Geometry: final body of the model. Coordinates: model frame, mm. A direction names the side the tool comes from. Give positions to 0.01 mm unless a question says otherwise; leave off trailing zeros. Loops run counter-clockwise (first coordinate to the right, second up) from the corner with the lowest first, then second, coordinate; pieces in that order, holes last. Notation, with made-up numbers: (-10.5, 65.5) - (42.5, 65.5) arc R19 ccw to (42.5, 101.5) - close; hole circle Ø5 at (-11.75, 54). An arc over 180 degrees is marked (long way). Use one line per item in the form item = value.
```python
from build123d import *

# Parameters (mm, degrees)
F0_W     = 6.35
F0_H     = 78.9432
F0_R     = 1.7145
F0_H_2   = 35.56
F1_DEPTH = 6.35
F2_DEPTH = 8.255


with BuildPart() as f1:
    # F0 (on Front) → F1 (new body)
    with BuildSketch(Plane.XZ):
        with Locations((-53.975, 30.3784)):
            Rectangle(F0_W, F0_H)
        with Locations((-53.975, -4.9657)):
            Circle(F0_R, mode=Mode.SUBTRACT)
        with Locations((-53.975, 65.7225)):
            Circle(F0_R, mode=Mode.SUBTRACT)
        with Locations((-53.975, -52.07)):
            Rectangle(F0_W, F0_H_2)
        with Locations((-53.975, -65.7225)):
            Circle(F0_R, mode=Mode.SUBTRACT)
        with Locations((-53.975, -38.4175)):
            Circle(F0_R, mode=Mode.SUBTRACT)
        with Locations((53.975, -52.07)):
            Rectangle(F0_W, F0_H_2)
        with Locations((53.975, -65.7225)):
            Circle(F0_R, mode=Mode.SUBTRACT)
        with Locations((53.975, -38.4175)):
            Circle(F0_R, mode=Mode.SUBTRACT)
        with Locations((53.975, 30.3784)):
            Rectangle(F0_W, F0_H)
        with Locations((53.975, -4.9657)):
            Circle(F0_R, mode=Mode.SUBTRACT)
        with Locations((53.975, 65.7225)):
            Circle(F0_R, mode=Mode.SUBTRACT)
        Polygon((-47.625, -69.85), (47.625, -69.85), (47.625, -31.115), (57.15, -31.115), (57.15, -12.2682), (47.625, -12.2682), (47.625, 69.85), (28.575, 69.85), (28.575, 31.75), (-28.575, 31.75), (-28.575, 69.85), (-47.625, 69.85), (-47.625, -12.2682), (-57.15, -12.2682), (-57.15, -31.115), (-47.625, -31.115), align=None)
        Polygon((-14.605, 15.875), (-14.605, 19.05), (-8.255, 19.05), (-8.255, 15.875), (-8.255, -38.2016), (-8.255, -41.3766), (-14.605, -41.3766), (-14.605, -38.2016), align=None, mode=Mode.SUBTRACT)
        Polygon((8.255, 15.875), (8.255, 19.05), (14.605, 19.05), (14.605, 15.875), (14.605, -38.2016), (14.605, -41.3766), (8.255, -41.3766), (8.255, -38.2016), align=None, mode=Mode.SUBTRACT)
    extrude(amount=F1_DEPTH)

    # F0 (on Front) → F2 (join)
    with BuildSketch(Plane.XZ):
        Polygon((47.625, -12.2682), (57.15, -12.2682), (57.15, -9.0932), (50.8, -9.0932), (50.8, 69.85), (47.625, 69.85), align=None)
        Polygon((47.625, -69.85), (50.8, -69.85), (50.8, -34.29), (57.15, -34.29), (57.15, -31.115), (47.625, -31.115), align=None)
        Polygon((-57.15, -9.0932), (-57.15, -12.2682), (-47.625, -12.2682), (-47.625, 69.85), (-50.8, 69.85), (-50.8, -9.0932), align=None)
        Polygon((-50.8, -69.85), (-47.625, -69.85), (-47.625, -31.115), (-57.15, -31.115), (-57.15, -34.29), (-50.8, -34.29), align=None)
    extrude(amount=F2_DEPTH)


solid = f1.part
```
(1) Cut plane A-A (z = 8). Return the cut outline in (x, y) (3 decimals), plus the area to 3 significant figures.
Solution:
outline = (-57.15, -6.35) - (-50.8, -6.35) - (-50.8, -8.255) - (-47.625, -8.255) - (-47.625, -6.35) - (-14.605, -6.35) - (-14.605, 0) - (-57.15, 0) - close; (-8.255, -6.35) - (8.255, -6.35) - (8.255, 0) - (-8.255, 0) - close; (14.605, -6.35) - (47.625, -6.35) - (47.625, -8.255) - (50.8, -8.255) - (50.8, -6.35) - (57.15, -6.35) - (57.15, 0) - (14.605, 0) - close
area = 657 mm2
(2) Access query for faces 1 (the face through (0, -3, 31.75)), 2 (the face through (11, -3, -41.377)), 3 (the face through (-54, -6.35, 31)). Directions: +Z, -Z, +X, -X, +Y, -Y. A direction counts if a zero-diameter tool reaches every point of the face in a straight line with its end or side. Return the directions, or none.
Solution:
face_1 = +Z, +Y, -Y
face_2 = +Y, -Y
face_3 = +Z, -X, -Y
(3) Material intervals for L1, parallel to X at y = -5.75, z = -1 (3 decimals); L2, parallel to X at y = -1, z = -5 (3 decimals); L3, parallel to X at y = -7.5, z = 15 (3 decimals), sorted ascending. Write a range as from..to.
Solution:
L1 = -57.15..-14.605, -8.255..8.255, 14.605..57.15
L2 = -57.15..-55.689, -52.261..-14.605, -8.255..8.255, 14.605..52.261, 55.689..57.15
L3 = -50.8..-47.625, 47.625..50.8
(4) Pin query (flat end, axial travel): P1, Ø4.5, axis at x = 53.98, z = 65.72, coming from the -Y side; P2, Ø6, axis at x = -31, z = 48, coming from the +Y side; P3, Ø0.6, axis at y = -7, z = -55, coming from the +X side; P4, Ø2, axis at x = 54, y = -7.5, coming from the +Z side. Return the tip coordinate at first contact, or that it passes through.
Solution:
P1 = -6.35
P2 = 0
P3 = 50.8
P4 = -9.09
(5) Cut plane B-B (x = -10.5). Return the cut outline in (y, z).
Solution:
outline = (-6.35, -69.85) - (0, -69.85) - (0, -41.38) - (-6.35, -41.38) - close; (-6.35, 19.05) - (0, 19.05) - (0, 31.75) - (-6.35, 31.75) - close
(6) Pull-direction query (Z, two-part tool) for faces 4 (the face through (-1, -3, -69.85)), 5 (the face through (54.897, -3.131, 67.168)), 6 (the face through (-50, -8.255, 26)); classes: released by +Z, released by -Z, zero draft, split by the parting line, or undercut.
Solution:
face_4 = released by -Z
face_5 = undercut
face_6 = zero draft
(7) Cut plane D-D (z = -55). Return the cut outline in (x, y) (3 decimals).
Solution:
outline = (-57.15, -6.35) - (-50.8, -6.35) - (-50.8, -8.255) - (-47.625, -8.255) - (-47.625, -6.35) - (47.625, -6.35) - (47.625, -8.255) - (50.8, -8.255) - (50.8, -6.35) - (57.15, -6.35) - (57.15, 0) - (-57.15, 0) - close
(8) Cut plane C-C (z = 43.5). Return the cut outline in (x, y) (3 decimals), plus the area to 3 significant figures.
Solution:
outline = (-57.15, -6.35) - (-50.8, -6.35) - (-50.8, -8.255) - (-47.625, -8.255) - (-47.625, -6.35) - (-28.575, -6.35) - (-28.575, 0) - (-57.15, 0) - close; (28.575, -6.35) - (47.625, -6.35) - (47.625, -8.255) - (50.8, -8.255) - (50.8, -6.35) - (57.15, -6.35) - (57.15, 0) - (28.575, 0) - close
area = 375 mm2
